Verification items for the finished model (mm, model axes). Face numbers are marked on the shaded views. A direction names the side the tool comes from. Give positions to 0.01 mm unless a question says otherwise; leave off trailing zeros. Loops run counter-clockwise (first coordinate to the right, second up) from the corner with the lowest first, then second, coordinate; pieces in that order, holes last. Notation, with made-up numbers: M -19.75,-0.75 L -4.75,-0.75 A10 ccw -4.75,13.25 Z; hole C 13.25,71.25 d7. An arc over 180 degrees is marked long. Answer in a Markdown table with one row per item.
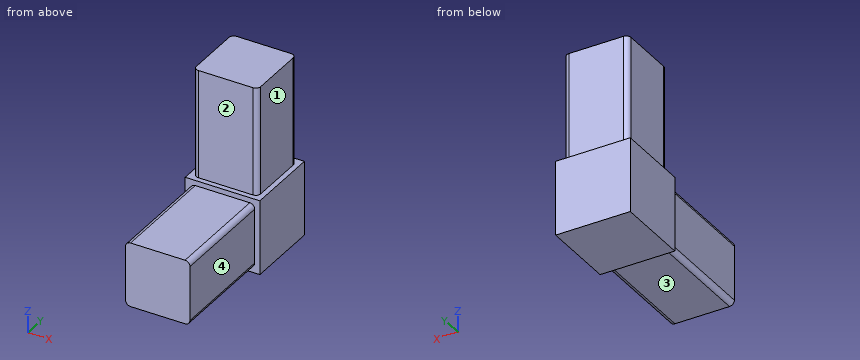
```python
from build123d import *

# Parameters (mm, degrees)
SKETCH1_W           = 16.637
SKETCH1_H           = 16.637
BOSS_EXTRUDE1_DEPTH = 28.067
SKETCH2_W           = 19.304
SKETCH2_H           = 19.304
BOSS_EXTRUDE2_DEPTH = 19.304
SKETCH3_W           = 16.637
SKETCH3_H           = 16.637
BOSS_EXTRUDE3_DEPTH = 28.067
FILLET1_R           = 1.27


with BuildPart() as part:
    # Sketch1 → Boss-Extrude1 (new body)
    with BuildSketch(Plane(origin=(0, 0, 0), x_dir=(1, 0, 0), z_dir=(0, 1, 0))):
        Rectangle(SKETCH1_W, SKETCH1_H)
    extrude(amount=BOSS_EXTRUDE1_DEPTH)

    # Sketch2 → Boss-Extrude2 (add)
    with BuildSketch(Plane(origin=(0, 28.067, 0), x_dir=(1, 0, 0), z_dir=(0, 1, 0))):
        Rectangle(SKETCH2_W, SKETCH2_H)
    extrude(amount=BOSS_EXTRUDE2_DEPTH)

    # Sketch3 → Boss-Extrude3 (add)
    with BuildSketch(Plane.XY.offset(9.652)):
        with Locations((0, 37.719)):
            Rectangle(SKETCH3_W, SKETCH3_H)
    extrude(amount=BOSS_EXTRUDE3_DEPTH)

    # Fillet1
    fillet1_edges = [part.edges().sort_by_distance(p)[0] for p in [
        (8.3185, 29.4005, 23.6855),
        (8.3185, 46.0375, 23.6855),
        (-8.3185, 46.0375, 23.6855),
        (-8.3185, 29.4005, 23.6855),
        (8.3185, 14.0335, 8.3185),
        (-8.3185, 14.0335, 8.3185),
        (-8.3185, 14.0335, -8.3185),
        (8.3185, 14.0335, -8.3185),
    ]]
    fillet(fillet1_edges, radius=FILLET1_R)


solid = part.part
```
Item 1: Sectioned sample at B-B (z = 17.5). Record the cut outline in (x, y).
Reported:
| item | result |
|---|---|
| outline | M -8.32,30.67 A1.27 ccw -7.05,29.4 L 7.05,29.4 A1.27 ccw 8.32,30.67 L 8.32,44.77 A1.27 ccw 7.05,46.04 L -7.05,46.04 A1.27 ccw -8.32,44.77 Z |
Item 2: Sectioned sample at D-D (z = 9). Record the cut outline in (x, y).
Reported:
| item | result |
|---|---|
| outline | M -9.65,28.07 L 9.65,28.07 L 9.65,47.37 L -9.65,47.37 Z |
Item 3: Go/stop test with flat-tipped pins: pin 1 (7 mm diameter, centred on y = 39.5, z = 22.5, fed in from +X); pin 2 (7 mm diameter, centred on x = -2, z = 24, fed in from -Y); pin 3 (1.5 mm diameter, centred on x = -1.5, y = 12, fed in from +Z). Record where each tip stops, or that it passes through.
Reported:
| item | result |
|---|---|
| pin 1 | stops at x = 8.32 |
| pin 2 | stops at y = 29.4 |
| pin 3 | stops at z = 8.32 |
Item 4: Sectioned sample at A-A (y = 9). Record the cut outline in (x, z).
Reported:
| item | result |
|---|---|
| outline | M -8.32,-7.05 A1.27 ccw -7.05,-8.32 L 7.05,-8.32 A1.27 ccw 8.32,-7.05 L 8.32,7.05 A1.27 ccw 7.05,8.32 L -7.05,8.32 A1.27 ccw -8.32,7.05 Z |
Item 5: Scan lines: L1, parallel to Y at x = -1, z = 22; L2, parallel to Z at x = -6.5, y = 24.5; L3, parallel to Z at x = 6.25, y = 29. Record each from-to range of solid material in increasing order. Write a range as [from, to].
Reported:
| item | result |
|---|---|
| L1 | y = [29.4, 46.04] |
| L2 | z = [-8.32, 8.32] |
| L3 | z = [-9.65, 9.65] |
Item 6: Sectioned sample at C-C (x = 2). Record the cut outline in (y, z), and give its area (3 significant figures).
Reported:
| item | result |
|---|---|
| outline | M 0,-8.32 L 28.07,-8.32 L 28.07,-9.65 L 47.37,-9.65 L 47.37,9.65 L 46.04,9.65 L 46.04,37.72 L 29.4,37.72 L 29.4,9.65 L 28.07,9.65 L 28.07,8.32 L 0,8.32 Z |
| area | 1,310 mm^2 |
Item 7: Tool access check on the marked faces 1, 2, 3 and 4. Record the directions out of +Z, -Z, +X, -X, +Y, -Y that give a thin tool (end or side, any length) a straight path to the whole face; none if there is none.
Reported:
| item | result |
|---|---|
| face 1 | +Z, +X, +Y, -Y |
| face 2 | +Z, +X, -X, -Y |
| face 3 | -Z, +X, -X, -Y |
| face 4 | +Z, -Z, +X, -Y |
